Geometry: final body of the model. Coordinates: model frame, mm. A direction names the side the tool comes from. Give positions to 0.01 mm unless a question says otherwise; leave off trailing zeros. Write each loop counter-clockwise with the first axis right and the second up, starting at its lowest first coordinate (ties: lowest second). Pieces come first, ordered by that corner, then holes.
```python
from build123d import *
from build123d.topology import SkipClean

# Parameters (mm, degrees)
ESQUISSE1_W                                        = 50.5
ESQUISSE1_H                                        = 51.7
ESQUISSE1_R                                        = 1.1
BOSS_EXTRU_1_DEPTH                                 = 3
CONG_1_R                                           = 1
CHAMBRAGE_POUR_VIS_SIX_PANS_CREUX_M1_6_D           = 2.2
CHAMBRAGE_POUR_VIS_SIX_PANS_CREUX_M1_6_CBORE_D     = 3.8
CHAMBRAGE_POUR_VIS_SIX_PANS_CREUX_M1_6_CBORE_DEPTH = 1.2
BOSS_EXTRU_2_START                                 = -19
ESQUISSE4_R                                        = 1.6
BOSS_EXTRU_2_DEPTH                                 = 19
ENL_V_START                                        = -19
ENL_V_MAT_EXTRU_1_DEPTH                            = 7
ENL_V_MAT_EXTRU_2_DEPTH                            = 77.075175977
ENL_V_MAT_EXTRU_2_DEPTH_BACK                       = 77.075175977
BOSS_EXTRU_3_DEPTH                                 = 2
CHANFREIN1_SIZE                                    = 2


with BuildPart() as part:
    # Esquisse1 → Boss.-Extru.1 (new body)
    with BuildSketch(Plane(origin=(0, 0, 0), x_dir=(1, 0, 0), z_dir=(0, 1, 0))):
        with Locations((4.2, -2.35)):
            Rectangle(ESQUISSE1_W, ESQUISSE1_H)
        with Locations(Location((-16.05, -25.2, 0), (0, 0, 270))):
            Circle(ESQUISSE1_R, mode=Mode.SUBTRACT)
        with Locations(Location((-16.05, -4.7, 0), (0, 0, 270))):
            Circle(ESQUISSE1_R, mode=Mode.SUBTRACT)
        with Locations(Location((8.4, -25.2, 0), (0, 0, 270))):
            Circle(ESQUISSE1_R, mode=Mode.SUBTRACT)
        with BuildLine():
            Line((-0.49, -5.46), (-0.49, -4.25))
            Line((-0.49, -4.25), (5.89, -4.25))
            Line((5.89, -4.25), (5.89, -11.085507795))
            ThreePointArc((5.89, -11.085507795), (18.661071136, -3.638740123), (28.18, -14.95))
            ThreePointArc((28.18, -14.95), (18.661071136, -26.261259877), (5.89, -18.814492205))
            Line((5.89, -18.814492205), (5.89, -25.65))
            Line((5.89, -25.65), (-0.49, -25.65))
            Line((-0.49, -25.65), (-0.49, -24.44))
            Line((-0.49, -24.44), (-13.14, -24.44))
            Line((-13.14, -24.44), (-13.14, -5.46))
            Line((-13.14, -5.46), (-0.49, -5.46))
        make_face(mode=Mode.SUBTRACT)
        with Locations(Location((8.4, -4.7, 0), (0, 0, 270))):
            Circle(ESQUISSE1_R, mode=Mode.SUBTRACT)
        with Locations(Location((0, 0, 0), (0, 0, 270))):
            Circle(ESQUISSE1_R, mode=Mode.SUBTRACT)
        with BuildLine():
            Line((8.89, 20.95), (8.89, 19.74))
            Line((8.89, 19.74), (21.54, 19.74))
            Line((21.54, 19.74), (21.54, 0.76))
            Line((21.54, 0.76), (8.89, 0.76))
            Line((8.89, 0.76), (8.89, -0.45))
            Line((8.89, -0.45), (2.51, -0.45))
            Line((2.51, -0.45), (2.51, 6.385507795))
            ThreePointArc((2.51, 6.385507795), (-19.78, 10.25), (2.51, 14.114492205))
            Line((2.51, 14.114492205), (2.51, 20.95))
            Line((2.51, 20.95), (8.89, 20.95))
        make_face(mode=Mode.SUBTRACT)
        with Locations(Location((0, 20.5, 0), (0, 0, 270))):
            Circle(ESQUISSE1_R, mode=Mode.SUBTRACT)
        with Locations(Location((24.45, 0, 0), (0, 0, 270))):
            Circle(ESQUISSE1_R, mode=Mode.SUBTRACT)
        with Locations(Location((24.45, 20.5, 0), (0, 0, 270))):
            Circle(ESQUISSE1_R, mode=Mode.SUBTRACT)
    extrude(amount=BOSS_EXTRU_1_DEPTH)

    # Congé1
    cong_1_edges = [part.edges().sort_by_distance(p)[0] for p in [
        (2.51, 1.5, -6.385507795),
        (2.51, 1.5, -14.114492205),
        (5.89, 1.5, 11.085507795),
        (5.89, 1.5, 18.814492205),
    ]]
    fillet(cong_1_edges, radius=CONG_1_R)

    # Chambrage pour vis à six pans creux M1.61 (through all)
    with Locations(Plane(origin=(0, 3, 0), x_dir=(1, 0, 0), z_dir=(0, 1, 0))):
        with Locations((-16.05, -4.7), (-16.05, -25.2), (8.4, -25.2), (8.4, -4.7), (0, 0), (0, 20.5), (24.45, 20.5), (24.45, 0)):
            CounterBoreHole(CHAMBRAGE_POUR_VIS_SIX_PANS_CREUX_M1_6_D / 2, CHAMBRAGE_POUR_VIS_SIX_PANS_CREUX_M1_6_CBORE_D / 2, CHAMBRAGE_POUR_VIS_SIX_PANS_CREUX_M1_6_CBORE_DEPTH)

    # Esquisse4 → Boss.-Extru.2 (add)
    # profile 1 of 2: a face of its own
    with SkipClean():  # the faces are left unmerged after this step: merging them gives an invalid solid
        with BuildSketch(Plane(origin=(0, 3, 0), x_dir=(1, 0, 0), z_dir=(0, 1, 0)).offset(BOSS_EXTRU_2_START)):
            with BuildLine():
                Line((-18.61, 23.5), (-30.21, 23.5))
                Line((-30.21, 23.5), (-30.21, -28.2))
                Line((-30.21, -28.2), (-18.61, -28.2))
                Line((-18.61, -28.2), (-18.61, 5.200811946))
                ThreePointArc((-18.61, 5.200811946), (-19.78, 10.25), (-18.61, 15.299188054))
                Line((-18.61, 15.299188054), (-18.61, 23.5))
            make_face()
            with Locations(Location((-24.41, 15.5, 0), (0, 0, 270))):
                Circle(ESQUISSE4_R, mode=Mode.SUBTRACT)
            with Locations(Location((-24.41, -20.2, 0), (0, 0, 90))):
                Circle(ESQUISSE4_R, mode=Mode.SUBTRACT)
        # profile 2 of 2: a face of its own
        with BuildSketch(Plane(origin=(0, 3, 0), x_dir=(1, 0, 0), z_dir=(0, 1, 0)).offset(BOSS_EXTRU_2_START)):
            with BuildLine():
                Line((27.01, 23.5), (38.61, 23.5))
                Line((38.61, 23.5), (38.61, -28.2))
                Line((38.61, -28.2), (27.01, -28.2))
                Line((27.01, -28.2), (27.01, -19.999188054))
                ThreePointArc((27.01, -19.999188054), (28.18, -14.95), (27.01, -9.900811946))
                Line((27.01, -9.900811946), (27.01, 23.5))
            make_face()
            with Locations(Location((32.81, 15.5, 0), (0, 0, 90))):
                Circle(ESQUISSE4_R, mode=Mode.SUBTRACT)
            with Locations(Location((32.81, -20.2, 0), (0, 0, 270))):
                Circle(ESQUISSE4_R, mode=Mode.SUBTRACT)
        extrude(amount=BOSS_EXTRU_2_DEPTH)

    # Esquisse5 → Enlèv. mat.-Extru.1 (cut)
    with SkipClean():  # the faces are left unmerged after this step: merging them gives an invalid solid
        with BuildSketch(Plane.XZ.offset(16).offset(ENL_V_START)):
            Polygon((-24.41, 23.433161507), (-27.21, 21.816580754), (-27.21, 18.583419246), (-24.41, 16.966838493), (-21.61, 18.583419246), (-21.61, 21.816580754), align=None)
            Polygon((-24.41, -12.266838493), (-27.21, -13.883419246), (-27.21, -17.116580754), (-24.41, -18.733161507), (-21.61, -17.116580754), (-21.61, -13.883419246), align=None)
            Polygon((32.81, -12.266838493), (30.01, -13.883419246), (30.01, -17.116580754), (32.81, -18.733161507), (35.61, -17.116580754), (35.61, -13.883419246), align=None)
            Polygon((32.81, 23.433161507), (30.01, 21.816580754), (30.01, 18.583419246), (32.81, 16.966838493), (35.61, 18.583419246), (35.61, 21.816580754), align=None)
        extrude(amount=ENL_V_MAT_EXTRU_1_DEPTH, mode=Mode.SUBTRACT)

    # Esquisse6 → Enlèv. mat.-Extru.2 (cut, two sides: drawn at the far end of the back side and taken through both)
    with SkipClean():  # the faces are left unmerged after this step: merging them gives an invalid solid
        with BuildSketch(Plane(origin=(38.61, 0, 0), x_dir=(0, 0, -1), z_dir=(1, 0, 0)).offset(-ENL_V_MAT_EXTRU_2_DEPTH_BACK)):
            Polygon((-28.2, -8.5), (-13.2, -8.5), (-7.35, -3), (2.65, -3), (8.5, -8.5), (23.5, -8.5), (23.5, -16), (-28.2, -16), align=None)
        extrude(amount=ENL_V_MAT_EXTRU_2_DEPTH + ENL_V_MAT_EXTRU_2_DEPTH_BACK, mode=Mode.SUBTRACT)

    # Esquisse7 → Boss.-Extru.3 (add)
    with SkipClean():  # the faces are left unmerged after this step: merging them gives an invalid solid
        with BuildSketch(Plane.XY.offset(28.2)):
            Polygon((-18.61, -8.5), (-14.205, -4.25), (22.605, -4.25), (27.01, -8.5), (38.61, -8.5), (38.61, 3), (-30.21, 3), (-30.21, -8.5), align=None)
        boss_extru_3 = extrude(amount=BOSS_EXTRU_3_DEPTH)

    # Symétrie1: Boss.-Extru.3 across plane
    with SkipClean():  # the faces are left unmerged after this step: merging them gives an invalid solid
        add(boss_extru_3.mirror(Plane.XY.offset(2.35)))

    # Chanfrein1
    chanfrein1_edges = [part.edges().sort_by_distance(p)[0] for p in [
        (-30.21, 3, 2.35),
        (38.61, 3, 2.35),
        (38.61, -2.75, 30.2),
        (4.2, 3, 30.2),
        (-30.21, -2.75, 30.2),
        (-30.21, -2.75, -25.5),
        (4.2, 3, -25.5),
        (38.61, -2.75, -25.5),
    ]]
    chamfer(chanfrein1_edges, length=CHANFREIN1_SIZE - 0.0001)  # a hair under: the kernel refuses the full size


solid = part.part
```
Item 1: Reachability of faces 4 (the face through (9, 1.8, 6)), 5 (the face through (-18.61, -4, -19)), 6 (the face through (-24.49, -5.71, -5.53)), 7 (the face through (6.547, 1.521, 21.725)) from +Z, -Z, +X, -X, +Y, -Y: full face, straight path, thin tool, end or side. Return the list, or none.
Found:
face 4: +Y
face 5: -Y
face 6: +X, -X, -Y
face 7: +Y, -Y
Item 2: Pull-direction query (Z, two-part tool) for faces 1 (the face through (1.853, 1.521, -17.025)), 2 (the face through (24.78, -6.35, 29.19)), 3 (the face through (-29.2, -3.68, 29.21)); classes: +Z half, -Z half, draft (parallel to the pull), parting line (faces both ways), or undercut.
Found:
face 1: undercut
face 2: draft
face 3: +Z half
Item 3: Section B-B, the plane x = 16.7. Return the cut outline in (y, z).
Found:
outline: (-4.25, -25.5) - (1, -25.5) - (3, -23.5) - (3, -19.74) - (0, -19.74) - (0, -23.5) - (-4.25, -23.5) - close; (-4.25, 28.2) - (0, 28.2) - (0, 26.43) - (3, 26.43) - (3, 28.2) - (1, 30.2) - (-4.25, 30.2) - close; (0, -0.76) - (3, -0.76) - (3, 3.47) - (0, 3.47) - close
Item 4: Section A-A, the plane z = 14.95. Return the cut outline in (x, y).
Found:
outline: (-30.21, -8.5) - (-18.61, -8.5) - (-18.61, 0) - (-13.14, 0) - (-13.14, 3) - (-28.21, 3) - (-30.21, 1) - close; (28.18, -8.5) - (38.61, -8.5) - (38.61, 1) - (36.61, 3) - (28.18, 3) - close
Item 5: Pin query (flat end, axial travel): pin 1 Ø4 at (x, z) = (-24.41, 20.2) entering from +Y; pin 2 Ø1.9 at (x, z) = (-16.5, 25.5) entering from +Y; pin 3 Ø5 at (x, z) = (15, -19.5) entering from -Y. Return the tip coordinate at first contact, or that it passes through.
Found:
pin 1: stops at y = -4
pin 2: stops at y = 1.8
pin 3: stops at y = 0
Item 6: Section D-D, the plane z = -9.5. Return the cut outline in (x, y).
Found:
outline: (-30.21, -8.5) - (-19.76, -8.5) - (-19.76, 3) - (-28.21, 3) - (-30.21, 1) - close; (21.54, 0) - (27.01, 0) - (27.01, -8.5) - (38.61, -8.5) - (38.61, 1) - (36.61, 3) - (21.54, 3) - close
Item 7: Section C-C, the plane x = 24.45. State how many separate pieces and enclosed holes the cut face has, plus the area to 3 significant figures.
Found:
separate pieces: 4
enclosed holes: 0
area: 119 mm2
Item 8: Line query: L1, parallel to X at y = -7.45, z = 20.2; L2, parallel to X at y = -2.75, z = 2; L3, parallel to Z at x = 9, y = 1.25. Output: solid intervals per line, ascending.
Found:
L1: x = -30.21 to -26.01, -22.81 to -18.61, 27.01 to 31.21, 34.41 to 38.61
L2: x = -30.21 to -18.61, 27.01 to 38.61
L3: z = -25.25 to -19.74, -0.76 to 3.78, 5.62 to 6.44, 23.46 to 24.28, 26.12 to 29.95
